Work out the finished part from the listing and answer in its coordinate system (mm). Give positions to 0.01 mm unless a question says otherwise; leave off trailing zeros.
Autodesk Inventor part; units mm, degrees
ref_plane "YZ Plane" through (0, 0, 0) normal (1, 0, 0) x (0, 1, 0)
ref_plane "XZ Plane" through (0, 0, 0) normal (0, 1, 0) x (-1, 0, 0)
ref_plane "XY Plane" through (0, 0, 0) normal (0, 0, 1) x (1, 0, 0)
sketch "Sketch3" plane through (0, 0, 0) normal (0, 1, 0) x (-1, 0, 0)
  line L0 (5, 0) -> (-140, 0)
  line L1 (-140, 0) -> (-140, -15)
  line L2 (-140, -15) -> (5, -15)
  line L3 (5, -15) -> (5, 0)
  dimension "d6" = 145
  dimension "d7" = 15
extrude "Plate1" add sketch "Sketch3" along normal blind 3
sketch "Sketch5" plane through (0, 0, 0) normal (0, -1, 0) x (1, 0, 0)
  line L0 (-5, 0) -> (140, 0)
  line L1 (-5, -15) -> (-5, 0)
  line L2 (140, -15) -> (-5, -15)
  line L3 (140, 0) -> (140, -15)
  line L4 (140, 0) -> (140, -15) construction
  line L5 (140, -7.5) -> (135, -7.5) construction
  line L6 (135, -7.5) -> (135, -12.5) construction
  line L7 (135, -12.5) -> (135, -2.5) construction
  line L8 (135, -2.5) -> (130, -2.5) construction
  line L9 (130, -2.5) -> (130, -12.5) construction
  circle A0 centre (135, -2.5) radius 1
  circle A1 centre (135, -12.5) radius 1
  circle A2 centre (130, -2.5) radius 1
  circle A3 centre (130, -12.5) radius 1
  point P0 (0, 0)
  dimension "d19" = 5
  dimension "d20" = 5
  dimension "d21" = 10
  dimension "d22" = 5
  dimension "d23" = 2
  dimension "d24" = 2
  dimension "d25" = 2
  dimension "d26" = 2
extrude "Extrusion2" cut sketch "Sketch5" against normal blind 10 contours A0 | A1 | A2 | A3
sketch "Sketch6" plane through (0, 0, 0) normal (0, -1, 0) x (1, 0, 0)
  point P0 (0, 0)
ref_plane "Work Plane1" through (67.5, 0, 0) normal (1, 0, 0) x (0, 0, -1)
mirror "Mirror1" about plane through (67.5, 0, 0) normal (1, 0, 0) of "Extrusion2"
fillet "Fillet1" radius 0.5 4 edges at (-5, 1.5, 0) (140, 1.5, 0) (140, 1.5, -15) (-5, 1.5, -15)
equation "\"d8\" = Thickness"
equation "\"BendRadius\" = Thickness"
equation "\"BendReliefWidth\" = Thickness"
equation "\"BendReliefDepth\" = 0.5 * Thickness"
equation "\"CornerReliefSize\" = 4 * Thickness"
equation "\"MinimumRemnant\" = 2 * Thickness"
equation "\"TransitionRadius\" = BendRadius"
equation "\"JacobiRadiusSize\" = Thickness"
equation "\"GapSize\" = Thickness"
properties part number "LaminaSoporteAccionadorF" material "Stainless Steel"
Item 1: Consider line 1 (Z direction, x = 135, y = 1); line 2 (X direction, y = 1.25, z = -13). Determine where each line is inside the solid, lowest interval first.
Item 2: A flat-ended cylindrical pin translates along its axis: pin 1 Ø1.2 at (x, z) = (130, -2.5) entering from -Y. Find the tip coordinate at first contact, or state that the pin passes through.
Item 3: Determine the mould class of faces 1 (the face through (69, 1, -15)), 2 (the face through (140, 1, -7)), 3 (the face through (-5, 1, -8)) for opening direction X: released by +X, released by -X, zero draft, split by the parting line, or undercut.
Ans:
1. line 1: z = -15 to -13.5, -11.5 to -3.5, -1.5 to 0
1. line 2: x = -5 to -0.87, 0.87 to 4.13, 5.87 to 129.13, 130.87 to 134.13, 135.87 to 140
2. pin 1: passes through
3. face 1: zero draft
3. face 2: released by +X
3. face 3: released by -X
